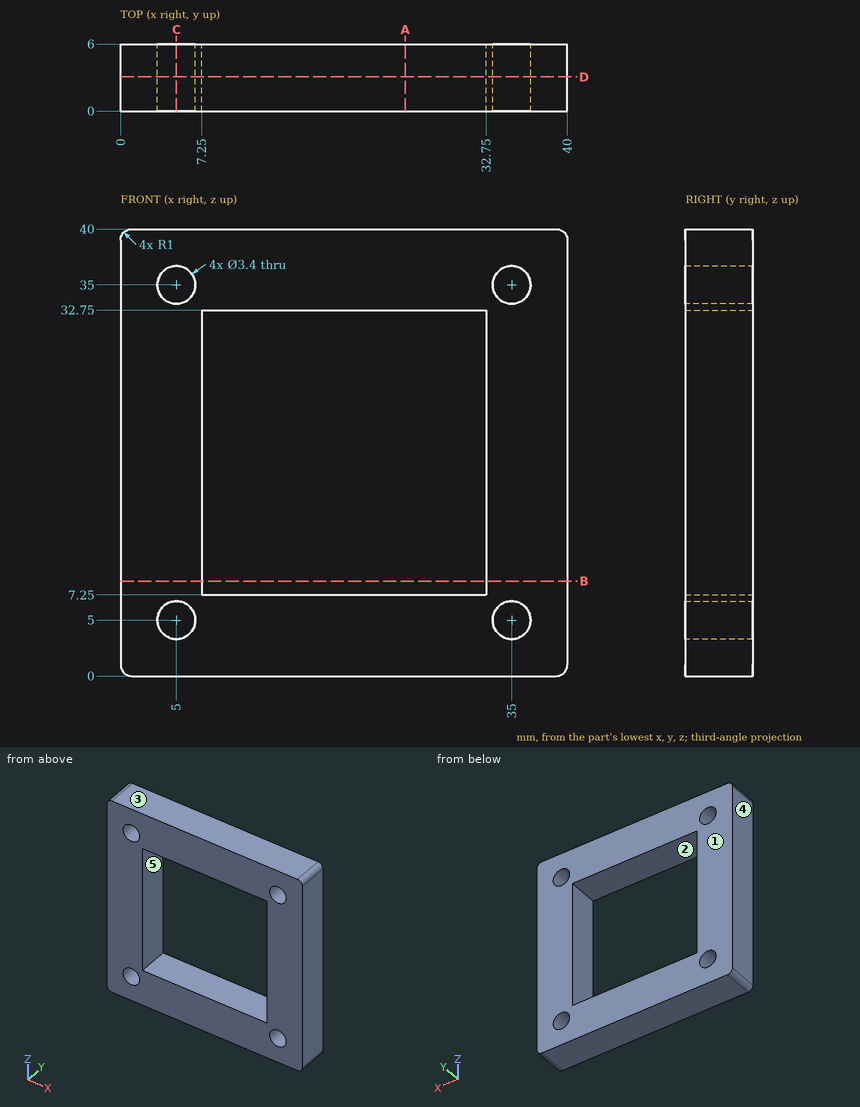
Verification items for this drawing (mm, ordinates from the low corner). A direction names the side the tool comes from. Give positions to 0.01 mm unless a question says otherwise; leave off trailing zeros. Write each loop counter-clockwise with the first axis right and the second up, starting at its lowest first coordinate (ties: lowest second). Pieces come first, ordered by that corner, then holes. Notation, with made-up numbers: (6, -30.75) - (62, -30.75) arc R20 cw to (62, -17.75) - close; hole circle Ø6 at (45, 6). An arc over 180 degrees is marked (long way). Answer as a JSON object with one key per item and string values. Group by question number.
1) Thickness scan on probe 1 along X at (y, z) = (3.35, 5); probe 2 along Z at (x, y) = (19.5, 3.9). Record the ranges inside material, lowest first. Write a range as from..to.
2) Sectioned sample at B-B (z = 8.5). Record the cut outline in (x, y), then the cut area to 3 significant figures.
3) Access from +Z, -Z, +X, -X, +Y, -Y to the whole of each face (thin tool, end or side, straight path). Record for the marked faces 1 and 2.
4) Sectioned sample at D-D (y = 3.05). Record the cut outline in (x, z), then the cut area to 3 significant figures.
5) Release check for a two-part mould opening along Z. For the marked faces 3, 4 and 5 record: pulls with the +Z half, pulls with the -Z half, needs draft (parallel to the pull), parting line crosses it, or undercut.
6) Sectioned sample at A-A (x = 25.5). Record the cut outline in (y, z).
7) Sectioned sample at C-C (x = 5). Record the cut outline in (y, z).
Geometry results:
{
 "1": {"probe 1": "x = 0..3.3, 6.7..33.3, 36.7..40", "probe 2": "z = 0..7.25, 32.75..40"},
 "2": {"outline": "(0, 0) - (7.25, 0) - (7.25, 6) - (0, 6) - close; (32.75, 0) - (40, 0) - (40, 6) - (32.75, 6) - close", "area": "87.0 mm^2"},
 "3": {"face 1": "+Z, -Z, +X, -X, +Y", "face 2": "+Y, -Y"},
 "4": {"outline": "(0, 1) arc R1 ccw to (1, 0) - (39, 0) arc R1 ccw to (40, 1) - (40, 39) arc R1 ccw to (39, 40) - (1, 40) arc R1 ccw to (0, 39) - close; hole circle Ø3.4 at (5, 5); hole circle Ø3.4 at (5, 35); hole (7.25, 7.25) - (32.75, 7.25) - (32.75, 32.75) - (7.25, 32.75) - close; hole circle Ø3.4 at (35, 5); hole circle Ø3.4 at (35, 35)", "area": "913 mm^2"},
 "5": {"face 3": "pulls with the +Z half", "face 4": "needs draft", "face 5": "undercut"},
 "6": {"outline": "(0, 0) - (6, 0) - (6, 7.25) - (0, 7.25) - close; (0, 32.75) - (6, 32.75) - (6, 40) - (0, 40) - close"},
 "7": {"outline": "(0, 0) - (6, 0) - (6, 3.3) - (0, 3.3) - close; (0, 6.7) - (6, 6.7) - (6, 33.3) - (0, 33.3) - close; (0, 36.7) - (6, 36.7) - (6, 40) - (0, 40) - close"}
}
